```python
from build123d import *

# Parameters (mm, degrees)
EXTRUDE_1_DEPTH          = 245
SKETCH_2_R               = 2
SKETCH_2_R_2             = 2.75
CUT_EXTRUDE_1_DEPTH      = 249.646335183
CUT_EXTRUDE_3_DEPTH      = 249.646335183
CUT_EXTRUDE_3_DEPTH_BACK = 249.646335183
SKETCH_4_R               = 2
CUT_EXTRUDE_4_DEPTH      = 249.646335183


with BuildPart() as part:
    # 草图1 → 凸台-拉伸1 (new, symmetric)
    with BuildSketch(Plane(origin=(0, 0, 0), x_dir=(1, 0, 0), z_dir=(0, 1, 0))):
        with BuildLine():
            Line((4, 0), (26, 0))
            ThreePointArc((26, 0), (28.828427125, 1.171572875), (30, 4))
            Line((30, 4), (30, 26))
            ThreePointArc((30, 26), (28.828427125, 28.828427125), (26, 30))
            Line((26, 30), (4, 30))
            ThreePointArc((4, 30), (1.171572875, 28.828427125), (0, 26))
            Line((0, 26), (0, 4))
            ThreePointArc((0, 4), (1.171572875, 1.171572875), (4, 0))
        make_face()
        with BuildLine():
            Line((4, 2), (26, 2))
            ThreePointArc((26, 2), (27.414213562, 2.585786438), (28, 4))
            Line((28, 4), (28, 26))
            ThreePointArc((28, 26), (27.414213562, 27.414213562), (26, 28))
            Line((26, 28), (4, 28))
            ThreePointArc((4, 28), (2.585786438, 27.414213562), (2, 26))
            Line((2, 26), (2, 4))
            ThreePointArc((2, 4), (2.585786438, 2.585786438), (4, 2))
        make_face(mode=Mode.SUBTRACT)
    extrude(amount=EXTRUDE_1_DEPTH, both=True)

    # 草图2 → 切除-拉伸1 (cut, through all)
    with BuildSketch(Plane(origin=(0, 0, 0), x_dir=(-1, 0, 0), z_dir=(0, 0, -1))):
        with Locations(Location((-22.5, 0, 0), (0, 0, 180))):
            Circle(SKETCH_2_R)
        with Locations(Location((-7.5, 0, 0), (0, 0, 180))):
            Circle(SKETCH_2_R)
        with Locations(Location((-15, 205, 0), (0, 0, 180))):
            Circle(SKETCH_2_R_2)
        with Locations(Location((-15, 71, 0), (0, 0, 180))):
            Circle(SKETCH_2_R_2)
        with Locations(Location((-15, -71, 0), (0, 0, 180))):
            Circle(SKETCH_2_R_2)
        with Locations(Location((-15, -205, 0), (0, 0, 180))):
            Circle(SKETCH_2_R_2)
    extrude(amount=CUT_EXTRUDE_1_DEPTH, mode=Mode.SUBTRACT)

    # 草图3 → 切除-拉伸3 (cut, two sides: drawn at the far end of the back side and taken through both)
    with BuildSketch(Plane(origin=(0, 0, 0), x_dir=(0, 0, -1), z_dir=(1, 0, 0)).offset(-CUT_EXTRUDE_3_DEPTH_BACK)):
        Polygon((30, 245), (0, 227.679491924), (0, 245), align=None)
        Polygon((0, -245), (30, -245), (0, -227.679491924), align=None)
    extrude(amount=CUT_EXTRUDE_3_DEPTH + CUT_EXTRUDE_3_DEPTH_BACK, mode=Mode.SUBTRACT)

    # 草图4 → 切除-拉伸4 (cut, through all)
    with BuildSketch(Plane(origin=(0, 0, 0), x_dir=(0, 0, -1), z_dir=(1, 0, 0))):
        with Locations(Location((15, 220, 0), (0, 0, 180))):
            Circle(SKETCH_4_R)
        with Locations(Location((15, 70, 0), (0, 0, 180))):
            Circle(SKETCH_4_R)
        with Locations(Location((15, -70, 0), (0, 0, 180))):
            Circle(SKETCH_4_R)
        with Locations(Location((15, -220, 0), (0, 0, 180))):
            Circle(SKETCH_4_R)
    extrude(amount=CUT_EXTRUDE_4_DEPTH, mode=Mode.SUBTRACT)


solid = part.part
```
Build history of the part. All positions in model axes, mm. A direction names the side the tool comes from. Coordinates: 2 decimals unless noted, no trailing zeros. Order: outer loops, then holes, each group sorted by start corner. A loop starts at its lowest first (then second) coordinate and runs counter-clockwise, first axis right, second up. Notation, with made-up numbers: M -2,74.25 L 19,74.25 A15 cw 19,84.25 Z; hole C 65.25,44.5 d10. An arc over 180 degrees is marked long. One line per question, with ' | ' between items. Start each with the question number.
1. Mould opens along Z. For faces 3 (the face through (0, 3, -15)), 4 (the face through (1.46, -236.46, -15.21)), 5 (the face through (28, 3, -15)) say: +Z half, -Z half, draft (parallel to the pull), parting line (faces both ways), or undercut.
2. Wall check: line 1 along X through (y, z) = (92.5, -21.75); line 2 along Z through (x, y) = (3.5, -84); line 3 along Y through (x, z) = (15, -28.7). Give the ranges that are in metal, low to high. Write a range as [from, to].
3. Flat gauge pins, fed straight in: P1, Ø5, axis at x = 19, z = -24, coming from the -Y side; P2, Ø12, axis at x = 26, z = -14.5, coming from the -Y side. Where does each tip first touch, or does it go through?
4. Cut at A-A (y = -62). Write the cut outline in (x, z).
5. Tool access for faces 1 (the face through (15, 3, -2)), 2 (the face through (30, 3, -15)): list every direction of +Z, -Z, +X, -X, +Y, -Y with a clear straight run to the whole face (end or side of a thin tool).
The answers:
1) face 3: draft | face 4: +Z half | face 5: undercut
2) line 1: x = [0, 2], [28, 30] | line 2: z = [-29.97, -27.94], [-2.06, -0.03] | line 3: y = [-244.25, -207.75], [-202.25, -73.75], [-68.25, 68.25], [73.75, 202.25], [207.75, 244.25]
3) P1: passes through | P2: stops at y = -239.32
4) outline: M 0,-26 A4 ccw 4,-30 L 26,-30 A4 ccw 30,-26 L 30,-4 A4 ccw 26,0 L 4,0 A4 ccw 0,-4 Z; hole M 2,-26 A2 ccw 4,-28 L 26,-28 A2 ccw 28,-26 L 28,-4 A2 ccw 26,-2 L 4,-2 A2 ccw 2,-4 Z
5) face 1: +Y, -Y | face 2: +Z, -Z, +X, +Y, -Y
